Geometry check sheet. Reference: the model listing, model coordinates, mm. Coordinates: 2 decimals unless noted, no trailing zeros. Loops run counter-clockwise (first coordinate to the right, second up) from the corner with the lowest first, then second, coordinate; pieces in that order, holes last.
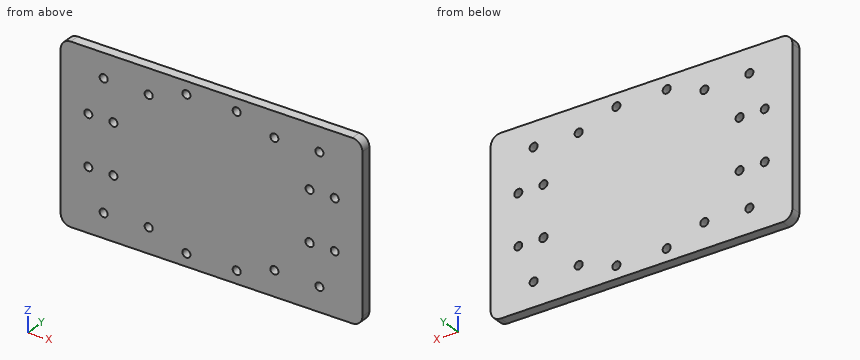
from build123d import *

# Parameters (mm, degrees)
SKETCH_1_W          = 120
SKETCH_1_H          = 70
EXTRUDE_1_DEPTH     = 4
SKETCH_2_R          = 1.6
SKETCH_2_R_2        = 1.55
SKETCH_2_R_3        = 1.65
CUT_EXTRUDE_1_DEPTH = 4
SKETCH_3_R          = 1.6
CUT_EXTRUDE_2_DEPTH = 4
FILLET_1_R          = 4


with BuildPart() as part:
    # 草图1 → 凸台-拉伸1 (new body)
    with BuildSketch(Plane(origin=(0, 0, 0), x_dir=(1, 0, 0), z_dir=(0, 1, 0))):
        with Locations((60, 35)):
            Rectangle(SKETCH_1_W, SKETCH_1_H)
    extrude(amount=EXTRUDE_1_DEPTH)

    # 草图2 → 切除-拉伸1 (cut)
    with BuildSketch(Plane(origin=(0, 4, 0), x_dir=(1, 0, 0), z_dir=(0, 1, 0))):
        with Locations(Location((11, 45, 0), (0, 0, 270))):
            Circle(SKETCH_2_R)
        with Locations(Location((21, 45, 0), (0, 0, 270))):
            Circle(SKETCH_2_R)
        with Locations(Location((21, 25, 0), (0, 0, 270))):
            Circle(SKETCH_2_R)
        with Locations(Location((11, 25, 0), (0, 0, 270))):
            Circle(SKETCH_2_R)
        with Locations(Location((109, 45, 0), (0, 0, 270))):
            Circle(SKETCH_2_R_2)
        with Locations(Location((99, 45, 0), (0, 0, 270))):
            Circle(SKETCH_2_R_3)
        with Locations(Location((109, 25, 0), (0, 0, 270))):
            Circle(SKETCH_2_R)
        with Locations(Location((99, 25, 0), (0, 0, 270))):
            Circle(SKETCH_2_R)
        with Locations(Location((102.9, 9.6, 0), (0, 0, 270))):
            Circle(SKETCH_2_R)
        with Locations(Location((17.1, 9.6, 0), (0, 0, 270))):
            Circle(SKETCH_2_R)
        with Locations(Location((17.1, 60.4, 0), (0, 0, 270))):
            Circle(SKETCH_2_R)
        with Locations(Location((102.9, 60.4, 0), (0, 0, 270))):
            Circle(SKETCH_2_R)
        with Locations(Location((85, 60, 0), (0, 0, 270))):
            Circle(SKETCH_2_R)
        with Locations(Location((85, 10, 0), (0, 0, 270))):
            Circle(SKETCH_2_R)
        with Locations(Location((35, 10, 0), (0, 0, 270))):
            Circle(SKETCH_2_R)
        with Locations(Location((35, 60, 0), (0, 0, 270))):
            Circle(SKETCH_2_R)
    extrude(amount=-CUT_EXTRUDE_1_DEPTH, mode=Mode.SUBTRACT)

    # 草图3 → 切除-拉伸2 (cut)
    with BuildSketch(Plane(origin=(0, 4, 0), x_dir=(1, 0, 0), z_dir=(0, 1, 0))):
        with Locations(Location((50, 5, 0), (0, 0, 270))):
            Circle(SKETCH_3_R)
        with Locations(Location((70, 5, 0), (0, 0, 270))):
            Circle(SKETCH_3_R)
        with Locations(Location((50, 65, 0), (0, 0, 270))):
            Circle(SKETCH_3_R)
        with Locations(Location((70, 65, 0), (0, 0, 270))):
            Circle(SKETCH_3_R)
    extrude(amount=-CUT_EXTRUDE_2_DEPTH, mode=Mode.SUBTRACT)

    # 圆角1
    fillet_1_edges = [part.edges().sort_by_distance(p)[0] for p in [
        (0, 2, -70),
        (120, 2, -70),
        (120, 2, 0),
        (0, 2, 0),
    ]]
    fillet(fillet_1_edges, radius=FILLET_1_R)


solid = part.part
1) Section check C-C on y = 2.45. Count the separate pieces of the cut face and the enclosed holes in it, and give its area (3 significant figures).
Data:
separate pieces: 1
enclosed holes: 20
area: 8,230 mm2
2) Section check D-D on z = -10. Record the cut outline in (x, y).
Data:
outline: (0, 0) - (15.55, 0) - (15.55, 4) - (0, 4) - close; (18.65, 0) - (33.4, 0) - (33.4, 4) - (18.65, 4) - close; (36.6, 0) - (83.4, 0) - (83.4, 4) - (36.6, 4) - close; (86.6, 0) - (101.35, 0) - (101.35, 4) - (86.6, 4) - close; (104.45, 0) - (120, 0) - (120, 4) - (104.45, 4) - close
3) Section check A-A on x = 21. Record the cut outline in (y, z).
Data:
outline: (0, -70) - (4, -70) - (4, -46.6) - (0, -46.6) - close; (0, -43.4) - (4, -43.4) - (4, -26.6) - (0, -26.6) - close; (0, -23.4) - (4, -23.4) - (4, 0) - (0, 0) - close
4) Material ranges on probe 1 along X at (y, z) = (2.75, -45); probe 2 along X at (y, z) = (2.1, -25); probe 3 along X at (y, z) = (1.3, -5), recorded low to high.
Data:
probe 1: x = 0 to 9.4, 12.6 to 19.4, 22.6 to 97.35, 100.65 to 107.45, 110.55 to 120
probe 2: x = 0 to 9.4, 12.6 to 19.4, 22.6 to 97.4, 100.6 to 107.4, 110.6 to 120
probe 3: x = 0 to 48.4, 51.6 to 68.4, 71.6 to 120
5) Section check B-B on z = -45. Record the cut outline in (x, y).
Data:
outline: (0, 0) - (9.4, 0) - (9.4, 4) - (0, 4) - close; (12.6, 0) - (19.4, 0) - (19.4, 4) - (12.6, 4) - close; (22.6, 0) - (97.35, 0) - (97.35, 4) - (22.6, 4) - close; (100.65, 0) - (107.45, 0) - (107.45, 4) - (100.65, 4) - close; (110.55, 0) - (120, 0) - (120, 4) - (110.55, 4) - close
6) Depth check by flat-ended pin: pin 1 (8 mm diameter, centred on x = 89.5, z = -53.5, fed in from -Y); pin 2 (1.9 mm diameter, centred on x = 17.1, z = -9.6, fed in from -Y). Enter the tip coordinate at first touch or a pass-through.
Data:
pin 1: stops at y = 0
pin 2: passes through
